```python
from build123d import *

# Parameters (mm, degrees)
MODEL_R             = 1.3
MODEL_R_2           = 3.6
BOSS_EXTRUDE1_DEPTH = 3


with BuildPart() as part:
    # Model → Boss-Extrude1 (new body)
    with BuildSketch(Plane.XY):
        with BuildLine():
            Line((54.4, 32.324975002), (54.4, 38.324975002))
            Line((54.4, 38.324975002), (56.5, 56.324876617))
            ThreePointArc((56.5, 56.324876617), (60.5, 60.324876617), (64.5, 56.324876617))
            Line((64.5, 56.324876617), (66.6, 38.324975002))
            Line((66.6, 38.324975002), (66.474361825, 25.879137217))
            ThreePointArc((66.474361825, 25.879137217), (60.71426202, 19.564875197), (54.4, 25.324975002))
            Line((54.4, 25.324975002), (54.4, 32.324975002))
        make_face()
        with Locations((60.5, 56.324876617)):
            Circle(MODEL_R, mode=Mode.SUBTRACT)
        with Locations((60.50005, 25.324984722)):
            Circle(MODEL_R_2, mode=Mode.SUBTRACT)
        with BuildLine():
            Line((59.5, 35.324934722), (59.5, 40.324934722))
            ThreePointArc((59.5, 40.324934722), (60.25, 41.074934722), (61, 40.324934722))
            Line((61, 40.324934722), (61, 35.324934722))
            ThreePointArc((61, 35.324934722), (60.25, 34.574934722), (59.5, 35.324934722))
        make_face(mode=Mode.SUBTRACT)
    extrude(amount=BOSS_EXTRUDE1_DEPTH)


solid = part.part
```
The listing builds one solid part. Answer for the finished solid, in the listing's coordinates (mm). A direction names the side the tool comes from. Give positions to 0.01 mm unless a question says otherwise; leave off trailing zeros. Order: outer loops, then holes, each group sorted by start corner. A loop starts at its lowest first (then second) coordinate and runs counter-clockwise, first axis right, second up.
1) For faces 1 (the face through (65.535, 47.451, 1.479)), 2 (the face through (61, 38, 1)), determine the directions among +Z, -Z, +X, -X, +Y, -Y from which every point of the face is accessible in a straight line to the end or side of a thin tool.
Reported:
face 1: +Z, -Z, +X, +Y
face 2: +Z, -Z
2) Find section A-A on z = 2.35. Write down the section's boundary in (x, y).
Reported:
outline: (54.4, 25.32) arc R6.04 ccw to (66.47, 25.88) - (66.6, 38.32) - (64.5, 56.32) arc R4 ccw to (56.5, 56.32) - (54.4, 38.32) - close; hole circle Ø7.2 at (60.5, 25.32); hole circle Ø2.6 at (60.5, 56.32); hole (59.5, 35.32) arc R0.75 ccw to (61, 35.32) - (61, 40.32) arc R0.75 ccw to (59.5, 40.32) - close
3) Consider line 1 along Y through (x, z) = (60.5, 2); line 2 along Y through (x, z) = (60.75, 2.4); line 3 along X through (y, z) = (56, 2.25). Determine where each line is inside the solid, lowest interval first.
Reported:
line 1: y = 19.56 to 21.72, 28.92 to 34.62, 41.03 to 55.02, 57.62 to 60.32
line 2: y = 19.57 to 21.73, 28.92 to 34.77, 40.88 to 55.05, 57.6 to 60.32
line 3: x = 56.46 to 59.24, 61.76 to 64.54
4) Find section D-D on y = 37.5. Write down the section's boundary in (x, z), then the cut area to 3 significant figures.
Reported:
outline: (54.4, 0) - (59.5, 0) - (59.5, 3) - (54.4, 3) - close; (61, 0) - (66.59, 0) - (66.59, 3) - (61, 3) - close
area: 32.1 mm2
5) Determine the mould class of faces 3 (the face through (60.234, 41.075, 1.479)), 4 (the face through (59, 40, 3)), 5 (the face through (60.266, 34.575, 1.479)), 6 (the face through (54.4, 32, 1)) for opening direction X: pulls with the +X half, pulls with the -X half, needs draft (parallel to the pull), parting line crosses it, or undercut.
Reported:
face 3: undercut
face 4: needs draft
face 5: undercut
face 6: pulls with the -X half
6) Find section C-C on x = 60.5. Write down the section's boundary in (y, z), then the cut area to 3 significant figures.
Reported:
outline: (19.56, 0) - (21.72, 0) - (21.72, 3) - (19.56, 3) - close; (28.92, 0) - (34.62, 0) - (34.62, 3) - (28.92, 3) - close; (41.03, 0) - (55.02, 0) - (55.02, 3) - (41.03, 3) - close; (57.62, 0) - (60.32, 0) - (60.32, 3) - (57.62, 3) - close
area: 73.7 mm2
7) Given P1, Ø1.6, axis at x = 60.5, y = 56.32, coming from the +Z side; P2, Ø0.9, axis at y = 37, z = 1.5, coming from the +X side; P3, Ø1, axis at x = 56.5, z = 2.5, coming from the -Y side, each flat-ended and moving along its own axis, determine where each tip first touches the part or whether it passes through.
Reported:
P1: passes through
P2: stops at x = 66.59
P3: stops at y = 20.63
8) Find section B-B on y = 27. Write down the section's boundary in (x, z), then the cut area to 3 significant figures.
Reported:
outline: (54.4, 0) - (57.31, 0) - (57.31, 3) - (54.4, 3) - close; (63.69, 0) - (66.49, 0) - (66.49, 3) - (63.69, 3) - close
area: 17.1 mm2
